Can you work these out from the drawing? Everything is in mm from the part's minimum corner. A direction names the side the tool comes from. Coordinates: 2 decimals unless noted, no trailing zeros. Loops run counter-clockwise (first coordinate to the right, second up) from the corner with the lowest first, then second, coordinate; pieces in that order, holes last. Notation, with made-up numbers: (-21.75, 4) -> (5.25, 4) arc R21 ccw to (5.25, 15) -> close; hole circle Ø7 at (-1, -8). An arc over 180 degrees is marked (long way). One line per question, with ' | ' between items.
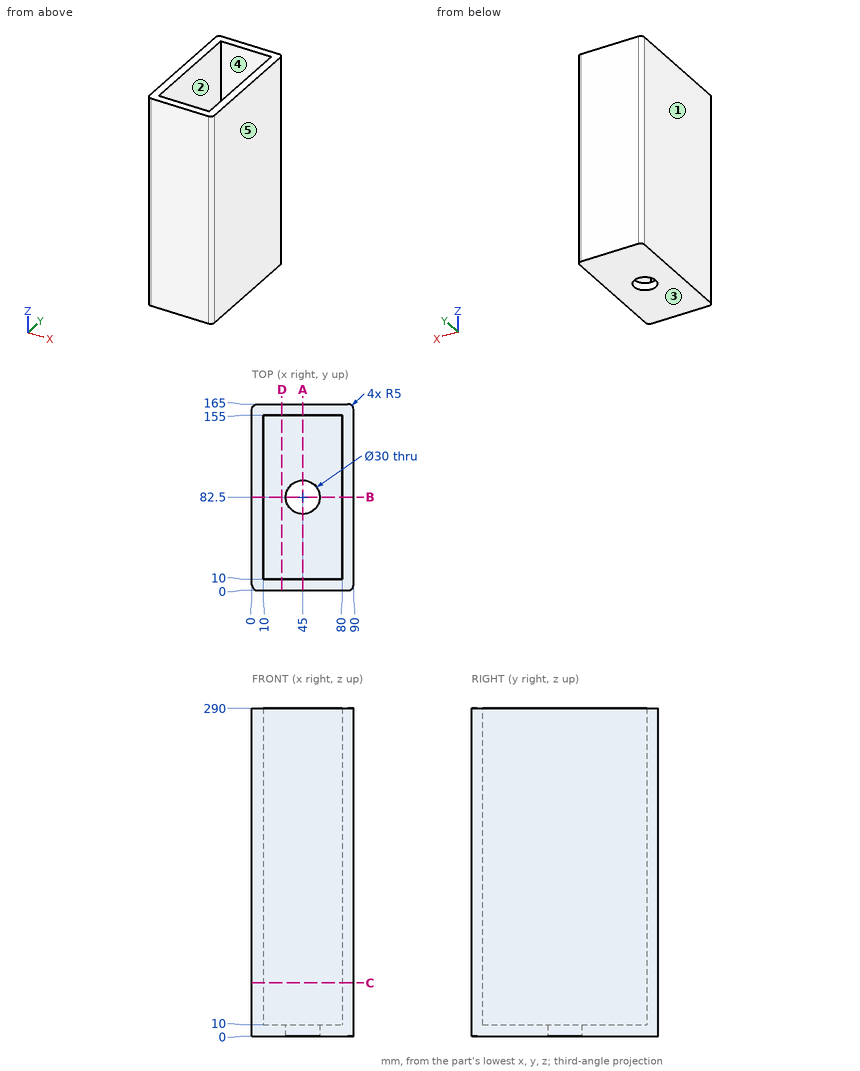
Q1. Please list where these lines run through material, in increasing order: L1, parallel to X at y = 122.5, z = 127; L2, parallel to Y at x = 29.5, z = 72.5; L3, parallel to Y at x = 45, z = 8. Write a range as [from, to].
Values follow:
L1: x = [0, 10], [80, 90] | L2: y = [0, 10], [155, 165] | L3: y = [0, 67.5], [97.5, 165]
Q2. Imagine slicing it at C-C on z = 47. Write out the boundary of the cut face in (x, y), plus the area to 3 significant figures.
Values follow:
outline: (0, 5) arc R5 ccw to (5, 0) -> (85, 0) arc R5 ccw to (90, 5) -> (90, 160) arc R5 ccw to (85, 165) -> (5, 165) arc R5 ccw to (0, 160) -> close; hole (10, 10) -> (80, 10) -> (80, 155) -> (10, 155) -> close | area: 4,680 mm2
Q3. We'd pull the mould along X, two halves only. Please class the marked faces 1, 2 and 3: released by +X, released by -X, zero draft, split by the parting line, or undercut.
Values follow:
face 1: released by -X | face 2: undercut | face 3: zero draft
Q4. Imagine slicing it at A-A on x = 45. Write out the boundary of the cut face in (y, z).
Values follow:
outline: (0, 0) -> (67.5, 0) -> (67.5, 10) -> (10, 10) -> (10, 290) -> (0, 290) -> close; (97.5, 0) -> (165, 0) -> (165, 290) -> (155, 290) -> (155, 10) -> (97.5, 10) -> close
Q5. Imagine slicing it at B-B on y = 82.5. Write out the boundary of the cut face in (x, z).
Values follow:
outline: (0, 0) -> (30, 0) -> (30, 10) -> (10, 10) -> (10, 290) -> (0, 290) -> close; (60, 0) -> (90, 0) -> (90, 290) -> (80, 290) -> (80, 10) -> (60, 10) -> close
Q6. Imagine slicing it at D-D on x = 26.5. Write out the boundary of the cut face in (y, z), plus the area to 3 significant figures.
Values follow:
outline: (0, 0) -> (165, 0) -> (165, 290) -> (155, 290) -> (155, 10) -> (10, 10) -> (10, 290) -> (0, 290) -> close | area: 7,250 mm2
Q7. For pin 1 (21 mm diameter, centred on x = 33, y = 80.5, fed in from +Z); pin 2 (1 mm diameter, centred on x = 69.5, z = 217, fed in from -Y), each with a flat end and sliding along its axis, tell me the tip position at first contact or that it passes through.
Values follow:
pin 1: stops at z = 10 | pin 2: stops at y = 0
Q8. For the marked faces 4 and 5, which set-ups out of +Z, -Z, +X, -X, +Y, -Y let a thin tool reach every point of the face, with its end or its side?
Values follow:
face 4: +Z | face 5: +Z, -Z, +X, +Y, -Y
